Read the model definition and answer for the solid it produces. Units are mm, in the model's axes. Give positions to 0.01 mm unless a question says otherwise; leave off trailing zeros. Order: outer loops, then holes, each group sorted by start corner. A loop starts at its lowest first (then second) coordinate and runs counter-clockwise, first axis right, second up. Notation, with made-up numbers: (72, -34.75) - (109, -34.75) arc R12 cw to (109, -21.75) - close; hole circle Ø11 at (83, 64.25). An arc over 180 degrees is marked (long way). Write item = value, one per line.
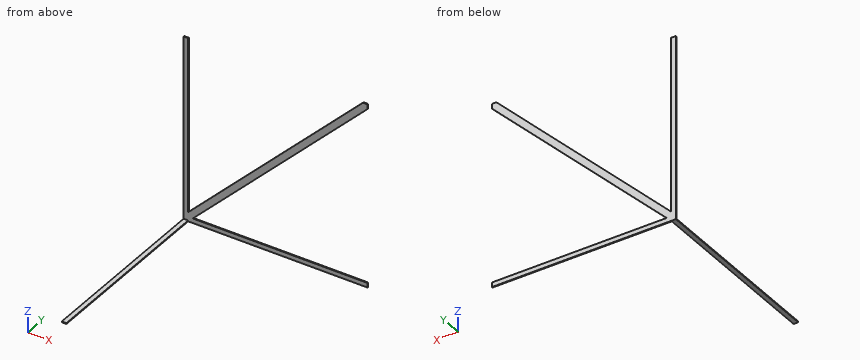
```python
from build123d import *

# Parameters (mm, degrees)
F1_DEPTH = 1
F2_W     = 5
F2_H     = 1
F3_DEPTH = 200


with BuildPart() as f1:
    # F0 (on Front) → F1 (new body)
    with BuildSketch(Plane.XZ):
        Polygon((0, 5), (0, 0), (5, 0), (200, 0), (200, 5), (10, 5), (200, 195), (200, 200), (195, 200), (5, 10), (5, 200), (0, 200), align=None)
    extrude(amount=F1_DEPTH)

    # F2 (on face) → F3 (join)
    with BuildSketch(Plane.XZ.offset(1)):
        with Locations((2.5, 0.5)):
            Rectangle(F2_W, F2_H)
    extrude(amount=F3_DEPTH)


solid = f1.part
```
1. Section C-C (y = -139) is taken. Determine the outline of the cut face in (x, z), and give its area (3 significant figures).
Recorded:
outline = (0, 0) - (5, 0) - (5, 1) - (0, 1) - close
area = 5.00 mm^2
2. A straight line is drawn through the part: L1, parallel to Y at x = 38.5, z = 41.5. Find the intervals that lie inside material, in ascending order. Write a range as [from, to].
Recorded:
L1 = [-1, 0]
3. Flat-ended cylindrical pins translate along their axes: pin 1 (1.1 mm diameter, centred on x = 63, y = -0.5, fed in from +Z); pin 2 (0.8 mm diameter, centred on y = -53, z = 0.5, fed in from +X); pin 3 (0.8 mm diameter, centred on y = -0.5, z = 103, fed in from +X). Find the tip coordinate at first contact, or state that the pin passes through.
Recorded:
pin_1 = 68.55
pin_2 = 5
pin_3 = 108.4
4. Section A-A (z = 122) is taken. Determine the outline of the cut face in (x, y), and give its area (3 significant figures).
Recorded:
outline = (0, -1) - (5, -1) - (5, 0) - (0, 0) - close; (117, -1) - (127, -1) - (127, 0) - (117, 0) - close
area = 15.0 mm^2
5. Section B-B (x = 156) is taken. Determine the outline of the cut face in (y, z).
Recorded:
outline = (-1, 0) - (0, 0) - (0, 5) - (-1, 5) - close; (-1, 151) - (0, 151) - (0, 161) - (-1, 161) - close
